The model under review builds one solid part; all positions refer to its coordinate system, in mm. A direction names the side the tool comes from. Round coordinates to 2 decimals unless told otherwise and drop trailing zeros. Write each loop counter-clockwise with the first axis right and the second up, starting at its lowest first coordinate (ties: lowest second). Pieces come first, ordered by that corner, then holes. Notation, with made-up numbers: (-37.5, 86.25) -> (-31.5, 86.25) arc R27 cw to (-31.5, 120.25) -> close; hole circle Ø2 at (22.25, 67). An arc over 180 degrees is marked (long way). Use CSV: the item, a comma, the result in double quotes. Start each with the question number.
1) Take a section at D-D, the plane y = 1.75. Give the boundary of the cut face in (x, z), then the cut area to 3 significant figures.
2) For pin 1 Ø10 at (x, z) = (-4, 5) entering from +Y; pin 2 Ø1 at (x, z) = (-13.75, -13) entering from -Y; pin 3 Ø1.3 at (x, z) = (13.75, 13) entering from +Y; pin 4 Ø2.5 at (x, z) = (-17, 0) entering from -Y, all flat-tipped, find the tip position at first contact; note any pin that passes through.
3) Wall thickness on probe 1 along Z at (x, y) = (-6, 7.25); probe 2 along Z at (x, y) = (-13.75, 7.55); probe 3 along X at (y, z) = (4.8, -13): over which ranges is each line inside the solid? List them lowest first. Write a range as [from, to].
4) Take a section at C-C, the plane x = -17. Give the boundary of the cut face in (y, z).
5) Take a section at A-A, the plane z = 0. Give the boundary of the cut face in (x, y).
6) Take a section at B-B, the plane y = 8. Give the boundary of the cut face in (x, z), then the cut area to 3 significant figures.
7) Mouldability with a two-part tool opening along Z and no side actions: class faces 1 (the face through (0, 0, -4)), 2 (the face through (18.1, 4.6, 11.6)), 3 (the face through (-9.43, 5.96, -14.4)) as released by +Z, released by -Z, zero draft, split by the parting line, or undercut.
8) Machinability: for faces 4 (the face through (0, 4, 17.3)), 5 (the face through (2, 3, 0)), which of the approach directions +Z, -Z, +X, -X, +Y, -Y give a long, thin tool a straight path to every point of the face, cutting with its end or side? Answer none if there is none.
from build123d import *

# Parameters (mm, degrees)
SKIZZE1_W                                            = 42
SKIZZE1_H                                            = 34.6
AUFSATZ_LINEAR_AUSTRAGEN1_DEPTH                      = 9
FORMSENKUNG_F_R_M3_SENKSCHRAUBE_MIT_SCHL_D           = 3.2
FORMSENKUNG_F_R_M3_SENKSCHRAUBE_MIT_SCHL_DEPTH       = 12.4
FORMSENKUNG_F_R_M3_SENKSCHRAUBE_MIT_SCHL_CSINK_D     = 6.3
FORMSENKUNG_F_R_M3_SENKSCHRAUBE_MIT_SCHL_CSINK_ANGLE = 90
FORMSENKUNG_F_R_M3_SENKSCHRAUBE_MIT_SCHL_TIP         = 0.96137699
SKIZZE17_W                                           = 20
SKIZZE17_H                                           = 30
SCHNITT_LINEAR_AUSTRAGEN2_DEPTH                      = 6
M2_GEWINDEBOHRUNG3_D                                 = 1.6
M2_GEWINDEBOHRUNG3_DEPTH                             = 6
M2_GEWINDEBOHRUNG3_CSINK_D                           = 2.05
M2_GEWINDEBOHRUNG3_CSINK_ANGLE                       = 90
M2_GEWINDEBOHRUNG3_TIP                               = 0.480688495
VERRUNDUNG2_R                                        = 2
F_3_0_3_DURCHMESSER_BOHRUNG3_D                       = 3
SCHNITT_LINEAR_AUSTRAGEN_D_NN1_DEPTH                 = 10
SCHNITT_LINEAR_AUSTRAGEN_D_NN1_DEPTH_BACK            = 10
SKIZZE24_R                                           = 31.5
SKIZZE24_R_2                                         = 21.5


with BuildPart() as part:
    # Skizze1 → Aufsatz-Linear austragen1 (new body)
    with BuildSketch(Plane(origin=(0, 0, 0), x_dir=(1, 0, 0), z_dir=(0, 1, 0))):
        Rectangle(SKIZZE1_W, SKIZZE1_H)
    extrude(amount=AUFSATZ_LINEAR_AUSTRAGEN1_DEPTH)

    # Formsenkung für M3 Senkschraube mit Schlitz/Kreuzschlitz1
    with Locations(Plane(origin=(0, 9, 0), x_dir=(1, 0, 0), z_dir=(0, 1, 0))):
        with Locations((-17, 0), (17, 0)):
            CounterSinkHole(FORMSENKUNG_F_R_M3_SENKSCHRAUBE_MIT_SCHL_D / 2, FORMSENKUNG_F_R_M3_SENKSCHRAUBE_MIT_SCHL_CSINK_D / 2, depth=FORMSENKUNG_F_R_M3_SENKSCHRAUBE_MIT_SCHL_DEPTH, counter_sink_angle=FORMSENKUNG_F_R_M3_SENKSCHRAUBE_MIT_SCHL_CSINK_ANGLE)
            with Locations((0, 0, -(FORMSENKUNG_F_R_M3_SENKSCHRAUBE_MIT_SCHL_DEPTH + FORMSENKUNG_F_R_M3_SENKSCHRAUBE_MIT_SCHL_TIP / 2))):  # 118° drill point
                Cone(0, FORMSENKUNG_F_R_M3_SENKSCHRAUBE_MIT_SCHL_D / 2, FORMSENKUNG_F_R_M3_SENKSCHRAUBE_MIT_SCHL_TIP, mode=Mode.SUBTRACT)

    # Skizze17 → Schnitt-Linear austragen2 (cut)
    with BuildSketch(Plane(origin=(0, 9, 0), x_dir=(1, 0, 0), z_dir=(0, 1, 0))):
        Rectangle(SKIZZE17_W, SKIZZE17_H)
    extrude(amount=-SCHNITT_LINEAR_AUSTRAGEN2_DEPTH, mode=Mode.SUBTRACT)

    # M2 Gewindebohrung3
    with Locations(Plane(origin=(0, 9, 0), x_dir=(1, 0, 0), z_dir=(0, 1, 0))):
        with Locations((-13.75, 13), (13.75, 13), (13.75, -13), (-13.75, -13)):
            CounterSinkHole(M2_GEWINDEBOHRUNG3_D / 2, M2_GEWINDEBOHRUNG3_CSINK_D / 2, depth=M2_GEWINDEBOHRUNG3_DEPTH, counter_sink_angle=M2_GEWINDEBOHRUNG3_CSINK_ANGLE)
            with Locations((0, 0, -(M2_GEWINDEBOHRUNG3_DEPTH + M2_GEWINDEBOHRUNG3_TIP / 2))):  # 118° drill point
                Cone(0, M2_GEWINDEBOHRUNG3_D / 2, M2_GEWINDEBOHRUNG3_TIP, mode=Mode.SUBTRACT)

    # Verrundung2
    verrundung2_edges = [part.edges().sort_by_distance(p)[0] for p in [
        (-10, 6, 15),
        (-10, 6, -15),
        (10, 6, -15),
        (10, 6, 15),
    ]]
    fillet(verrundung2_edges, radius=VERRUNDUNG2_R)

    # Ø3.0 (3) Durchmesser Bohrung3 (through all)
    with Locations(Plane(origin=(0, 3, 0), x_dir=(1, 0, 0), z_dir=(0, 1, 0))):
        with Locations((0, 0)):
            Hole(F_3_0_3_DURCHMESSER_BOHRUNG3_D / 2)

    # Skizze24 → Schnitt-Linear-Austragen-Dünn1 (cut, two sides: drawn at the far end of the back side and taken through both)
    with BuildSketch(Plane.XZ.offset(-SCHNITT_LINEAR_AUSTRAGEN_D_NN1_DEPTH_BACK)):
        Circle(SKIZZE24_R)
        Circle(SKIZZE24_R_2, mode=Mode.SUBTRACT)
    extrude(amount=SCHNITT_LINEAR_AUSTRAGEN_D_NN1_DEPTH + SCHNITT_LINEAR_AUSTRAGEN_D_NN1_DEPTH_BACK, mode=Mode.SUBTRACT)


solid = part.part
Values found:
1,outline,"(-21, -4.61) arc R21.5 ccw to (-12.77, -17.3) -> (12.77, -17.3) arc R21.5 ccw to (21, -4.61) -> (21, 4.61) arc R21.5 ccw to (12.77, 17.3) -> (-12.77, 17.3) arc R21.5 ccw to (-21, 4.61) -> close; hole circle Ø3.2 at (-17, 0); hole circle Ø3 at (0, 0); hole circle Ø3.2 at (17, 0)"
1,area,"1,280 mm²"
2,pin 1,"y = 3"
2,pin 2,"y = 0"
2,pin 3,"y = 2.91"
2,pin 4,"through"
3,probe 1,"[-17.3, -15], [15, 17.3]"
3,probe 2,"[-16.53, -13.8], [-12.2, 12.2], [13.8, 16.53]"
3,probe 3,"[-17.12, -14.55], [-12.95, -10], [10, 12.95], [14.55, 17.12]"
4,outline,"(0, -13.16) -> (9, -13.16) -> (9, -3.15) -> (7.45, -1.6) -> (0, -1.6) -> close; (0, 1.6) -> (7.45, 1.6) -> (9, 3.15) -> (9, 13.16) -> (0, 13.16) -> close"
5,outline,"(-21, 0) -> (-18.6, 0) -> (-18.6, 7.45) -> (-20.15, 9) -> (-21, 9) -> close; (-15.4, 0) -> (-1.5, 0) -> (-1.5, 3) -> (-10, 3) -> (-10, 9) -> (-13.85, 9) -> (-15.4, 7.45) -> close; (1.5, 0) -> (15.4, 0) -> (15.4, 7.45) -> (13.85, 9) -> (10, 9) -> (10, 3) -> (1.5, 3) -> close; (18.6, 0) -> (21, 0) -> (21, 9) -> (20.15, 9) -> (18.6, 7.45) -> close"
6,outline,"(-21, -4.61) arc R21.5 ccw to (-12.77, -17.3) -> (12.77, -17.3) arc R21.5 ccw to (21, -4.61) -> (21, 4.61) arc R21.5 ccw to (12.77, 17.3) -> (-12.77, 17.3) arc R21.5 ccw to (-21, 4.61) -> close; hole circle Ø4.3 at (-17, 0); hole circle Ø1.6 at (-13.75, -13); hole circle Ø1.6 at (-13.75, 13); hole (-10, -13) arc R2 ccw to (-8, -15) -> (8, -15) arc R2 ccw to (10, -13) -> (10, 13) arc R2 ccw to (8, 15) -> (-8, 15) arc R2 ccw to (-10, 13) -> close; hole circle Ø1.6 at (13.75, -13); hole circle Ø1.6 at (13.75, 13); hole circle Ø4.3 at (17, 0)"
6,area,"666 mm²"
7,face 1,"zero draft"
7,face 2,"released by +Z"
7,face 3,"undercut"
8,face 4,"+Z, +X, -X, +Y, -Y"
8,face 5,"+Y"
